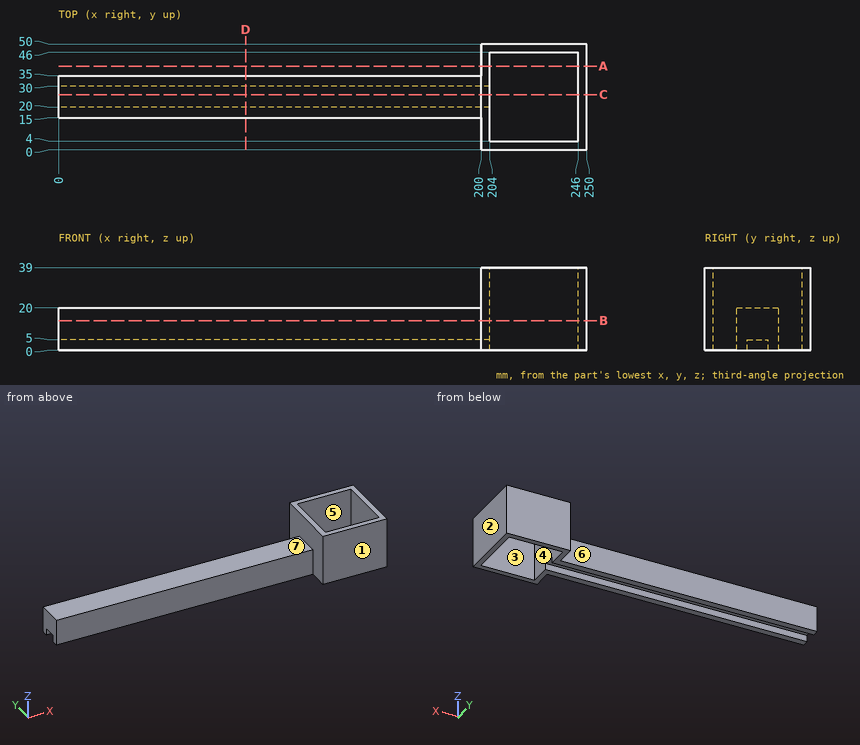
The drawing under review shows one solid part. Ordinate dimensions are in mm from its lowest x, y, z. A direction names the side the tool comes from. Coordinates: 2 decimals unless noted, no trailing zeros. Order: outer loops, then holes, each group sorted by start corner. A loop starts at its lowest first (then second) coordinate and runs counter-clockwise, first axis right, second up. Notation, with made-up numbers: (53, 47.25) -> (98, 47.25) arc R31 ccw to (98, 79.25) -> close; hole circle Ø5 at (-5.75, 20.25). An arc over 180 degrees is marked (long way). Answer in a Markdown table with one row per item. Add a question column.
Item 1: We need section A-A on y = 39.5. Write out the cut boundary in (x, z).
Item 2: Mouldability with a two-part tool opening along X and no side actions: class the marked faces 1, 2, 3 and 4 as +X half, -X half, draft (parallel to the pull), parting line (faces both ways), or undercut.
Item 3: Clearance check with flat-ended pins moving along their axes: pin 1 (6 mm diameter, centred on x = 35.5, y = 25.5, fed in from +Z); pin 2 (2.5 mm diameter, centred on x = 120.5, z = 2.5, fed in from +Y); pin 3 (2 mm diameter, centred on x = 41, y = 25, fed in from -Z). State where each tip first meets the part, or that it passes through.
Item 4: To check wall thickness, follow probe 1 along X at (y, z) = (13.5, 8.5); probe 2 along Y at (x, z) = (147, 3); probe 3 along X at (y, z) = (17, 10.5). State the ranges of each line that lie inside material, in increasing order.
Item 5: We need section B-B on z = 14. Write out the cut boundary in (x, y).
Item 6: Machinability: for the marked faces 5, 6 and 7, which of the approach directions +Z, -Z, +X, -X, +Y, -Y give a long, thin tool a straight path to every point of the face, cutting with its end or side? Answer none if there is none.
Item 7: We need section D-D on x = 88.5. Write out the cut boundary in (y, z), plus the area to 3 significant figures.
Item 8: We need section C-C on y = 26. Write out the cut boundary in (x, z).
Final values:
| question | item | result |
|---|---|---|
| 1 | outline | (200, 0) -> (204, 0) -> (204, 39) -> (200, 39) -> close; (246, 0) -> (250, 0) -> (250, 39) -> (246, 39) -> close |
| 2 | face 1 | draft |
| 2 | face 2 | +X half |
| 2 | face 3 | undercut |
| 2 | face 4 | undercut |
| 3 | pin 1 | stops at z = 20 |
| 3 | pin 2 | stops at y = 35 |
| 3 | pin 3 | stops at z = 5 |
| 4 | probe 1 | x = 200 to 204, 246 to 250 |
| 4 | probe 2 | y = 15 to 20, 30 to 35 |
| 4 | probe 3 | x = 0 to 204, 246 to 250 |
| 5 | outline | (0, 15) -> (200, 15) -> (200, 0) -> (250, 0) -> (250, 50) -> (200, 50) -> (200, 35) -> (0, 35) -> close; hole (204, 4) -> (246, 4) -> (246, 46) -> (204, 46) -> close |
| 6 | face 5 | +Z, -Z |
| 6 | face 6 | +Z, -Z, -X, +Y |
| 6 | face 7 | +Z, -X, +Y, -Y |
| 7 | outline | (15, 0) -> (20, 0) -> (20, 5) -> (30, 5) -> (30, 0) -> (35, 0) -> (35, 20) -> (15, 20) -> close |
| 7 | area | 350 mm2 |
| 8 | outline | (0, 5) -> (204, 5) -> (204, 39) -> (200, 39) -> (200, 20) -> (0, 20) -> close; (246, 0) -> (250, 0) -> (250, 39) -> (246, 39) -> close |
